```python
from build123d import *

# Parameters (mm, degrees)
SKETCH1_W            = 350
SKETCH1_H            = 150
BOSS_EXTRUDE1_DEPTH  = 5
SKETCH2_W            = 55
SKETCH2_H            = 42
BOSS_EXTRUDE2_DEPTH  = 5
SKETCH3_R            = 5
CUT_EXTRUDE1_DEPTH   = 225.138350132
FILLET1_R            = 20
FILLET1_OF_MIRROR1_R = 20
SKETCH5_R            = 5
CUT_EXTRUDE3_DEPTH   = 194.956180618
SKETCH6_R            = 5
CUT_EXTRUDE4_DEPTH   = 194.956180618


with BuildPart() as part:
    # Sketch1 → Boss-Extrude1 (new body)
    with BuildSketch(Plane(origin=(0, 0, 0), x_dir=(1, 0, 0), z_dir=(0, 1, 0))):
        Rectangle(SKETCH1_W, SKETCH1_H)
    extrude(amount=BOSS_EXTRUDE1_DEPTH)

    # Sketch2 → Boss-Extrude2 (add)
    with BuildSketch(Plane(origin=(27, 0, 0), x_dir=(0, 0, -1), z_dir=(1, 0, 0))):
        with Locations((-34.6, 21)):
            Rectangle(SKETCH2_W, SKETCH2_H)
    boss_extrude2 = extrude(amount=BOSS_EXTRUDE2_DEPTH)

    # Sketch3 → Cut-Extrude1 (cut, through all)
    with BuildSketch(Plane(origin=(32, 0, 0), x_dir=(0, 0, -1), z_dir=(1, 0, 0))):
        with Locations((-34.6, 30)):
            Circle(SKETCH3_R)
    cut_extrude1 = extrude(amount=-CUT_EXTRUDE1_DEPTH, mode=Mode.SUBTRACT)

    # Fillet1
    fillet1_edges = [part.edges().sort_by_distance(p)[0] for p in [
        (29.5, 42, 62.1),
        (29.5, 42, 7.1),
    ]]
    fillet(fillet1_edges, radius=FILLET1_R)

    # Mirror1: Boss-Extrude2, Cut-Extrude1 across plane
    add(boss_extrude2.mirror(Plane(origin=(0, 0, 0), x_dir=(0, 0, 1), z_dir=(1, 0, 0))))
    add(cut_extrude1.mirror(Plane(origin=(0, 0, 0), x_dir=(0, 0, 1), z_dir=(1, 0, 0))), mode=Mode.SUBTRACT)

    # Fillet1 of Mirror1
    fillet1_of_mirror1_edges = [part.edges().sort_by_distance(p)[0] for p in [
        (-29.5, 42, 62.1),
        (-29.5, 42, 7.1),
    ]]
    fillet(fillet1_of_mirror1_edges, radius=FILLET1_OF_MIRROR1_R)

    # Sketch5 → Cut-Extrude3 (cut, through all)
    with BuildSketch(Plane(origin=(0, 5, 0), x_dir=(1, 0, 0), z_dir=(0, 1, 0))):
        with Locations(Location((-55, 48.1, 0), (0, 0, 270))):
            Circle(SKETCH5_R)
        with Locations(Location((-55, 22.1, 0), (0, 0, 270))):
            Circle(SKETCH5_R)
    cut_extrude3 = extrude(amount=-CUT_EXTRUDE3_DEPTH, mode=Mode.SUBTRACT)

    # Mirror3: Cut-Extrude3 across plane
    add(cut_extrude3.mirror(Plane(origin=(0, 0, 0), x_dir=(0, 0, 1), z_dir=(1, 0, 0))), mode=Mode.SUBTRACT)

    # Sketch6 → Cut-Extrude4 (cut, through all)
    with BuildSketch(Plane(origin=(0, 5, 0), x_dir=(1, 0, 0), z_dir=(0, 1, 0))):
        with Locations(Location((-165, 60, 0), (0, 0, 270))):
            Circle(SKETCH6_R)
        with Locations(Location((-165, 20, 0), (0, 0, 270))):
            Circle(SKETCH6_R)
        with Locations(Location((-165, -20, 0), (0, 0, 270))):
            Circle(SKETCH6_R)
        with Locations(Location((-165, -60, 0), (0, 0, 270))):
            Circle(SKETCH6_R)
    cut_extrude4 = extrude(amount=-CUT_EXTRUDE4_DEPTH, mode=Mode.SUBTRACT)

    # Mirror4: Cut-Extrude4 across plane
    add(cut_extrude4.mirror(Plane(origin=(0, 0, 0), x_dir=(0, 0, 1), z_dir=(1, 0, 0))), mode=Mode.SUBTRACT)


solid = part.part
```
Geometry check sheet. Reference: the model listing, model coordinates, mm. A direction names the side the tool comes from. Give positions to 0.01 mm unless a question says otherwise; leave off trailing zeros. Order: outer loops, then holes, each group sorted by start corner. A loop starts at its lowest first (then second) coordinate and runs counter-clockwise, first axis right, second up. Notation, with made-up numbers: (-0.75, 63) -> (17.25, 63) arc R37 ccw to (17.25, 102) -> close; hole circle Ø2 at (-17, -10). An arc over 180 degrees is marked (long way). Write each question's results on one line, items separated by ' | '. Start each with the question number.
(1) Sectioned sample at A-A (x = -55). Enter the section's corners in (y, z), plus the area to 3 significant figures.
(2) Sectioned sample at D-D (z = 58.5). Enter the section's corners in (x, y).
(3) Sectioned sample at B-B (z = -60). Enter the section's corners in (x, y), plus the area to 3 significant figures.
(4) Mould release check, pull along Z, two halves, no side actions. Record for faces 5 (the face through (-29.535, 35.986, 12.803)), 6 (the face through (29.535, 35.986, 56.397)), 7 (the face through (-50.043, 2.535, -22.751)), 8 (the face through (-2, 5, -1)): pulls with the +Z half, pulls with the -Z half, needs draft (parallel to the pull), parting line crosses it, or undercut.
(5) Sectioned sample at C-C (y = 30). Enter the section's corners in (x, z), plus the area to 3 significant figures.
(6) Access from +Z, -Z, +X, -X, +Y, -Y to the whole of each face (thin tool, end or side, straight path). Record for faces 1 (the face through (-32, 24, 35)), 2 (the face through (-51.621, 2.535, -51.785)), 3 (the face through (27, 24, 35)), 4 (the face through (32, 24, 35)).
(7) Gauge pin test, flat ends, axial feed: P1, Ø1.5, axis at x = 28.5, y = 9.5, coming from the +Z side; P2, Ø5.5, axis at x = -30, y = 13.5, coming from the -Z side; P3, Ø11, axis at y = 16.5, z = 30, coming from the +X side. Record the tip position at first contact, or that the pin passes through.
(8) Scan lines: line 1 (Z direction, x = 165, y = 2.8); line 2 (X direction, y = 2.25, z = -48.1); line 3 (X direction, y = 3.6, z = -20). Record each from-to range of solid material in increasing order.
Answer below:
1) outline: (0, -75) -> (5, -75) -> (5, -53.1) -> (0, -53.1) -> close; (0, -43.1) -> (5, -43.1) -> (5, -27.1) -> (0, -27.1) -> close; (0, -17.1) -> (5, -17.1) -> (5, 75) -> (0, 75) -> close | area: 650 mm2
2) outline: (-175, 0) -> (-169.77, 0) -> (-169.77, 5) -> (-175, 5) -> close; (-160.23, 0) -> (160.23, 0) -> (160.23, 5) -> (32, 5) -> (32, 33.45) -> (27, 33.45) -> (27, 5) -> (-27, 5) -> (-27, 33.45) -> (-32, 33.45) -> (-32, 5) -> (-160.23, 5) -> close; (169.77, 0) -> (175, 0) -> (175, 5) -> (169.77, 5) -> close
3) outline: (-175, 0) -> (-170, 0) -> (-170, 5) -> (-175, 5) -> close; (-160, 0) -> (160, 0) -> (160, 5) -> (-160, 5) -> close; (170, 0) -> (175, 0) -> (175, 5) -> (170, 5) -> close | area: 1,650 mm2
4) face 5: pulls with the -Z half | face 6: pulls with the +Z half | face 7: undercut | face 8: needs draft
5) outline: (-32, 8.77) -> (-27, 8.77) -> (-27, 29.6) -> (-32, 29.6) -> close; (-32, 39.6) -> (-27, 39.6) -> (-27, 60.43) -> (-32, 60.43) -> close; (27, 8.77) -> (32, 8.77) -> (32, 29.6) -> (27, 29.6) -> close; (27, 39.6) -> (32, 39.6) -> (32, 60.43) -> (27, 60.43) -> close | area: 417 mm2
6) face 1: +Z, -Z, -X, +Y | face 2: +Y, -Y | face 3: +Z, -Z, +Y | face 4: +Z, -Z, +X, +Y
7) P1: z = 62.1 | P2: z = 7.1 | P3: x = 32
8) line 1: -75 to -65, -55 to -25, -15 to 15, 25 to 55, 65 to 75 | line 2: -175 to -60, -50 to 50, 60 to 175 | line 3: -175 to -170, -160 to -59.54, -50.46 to 50.46, 59.54 to 160, 170 to 175
